The listing builds one solid part. Answer for the finished solid, in the listing's coordinates (mm). Face numbers are marked on the shaded views. A direction names the side the tool comes from. Coordinates: 2 decimals unless noted, no trailing zeros. Order: outer loops, then holes, each group sorted by start corner. A loop starts at its lowest first (then second) coordinate and runs counter-clockwise, first axis right, second up. Notation, with made-up numbers: (87, -29) -> (145, -29) arc R17 ccw to (145, -6) -> close; hole circle Ø9 at (4.5, 72.5). An arc over 180 degrees is marked (long way). Write each question's results on one line, items separated by ' | '. Start each with the question number.
(1) The part is cut by section D-D, the plane x = 6. Give the vertices of the cut face in (y, z).
(2) The part is cut by section A-A, the plane y = 0. Give the vertices of the cut face in (x, z), then the cut area to 3 significant figures.
(3) A tool of negligible diameter and unlimited length cuts with its end or side. For the marked faces 1 and 2, from which of +Z, -Z, +X, -X, +Y, -Y can it reach the whole face along a straight path? Write none if from no direction.
(4) The part is cut by section C-C, the plane z = 3.5. Give the vertices of the cut face in (x, y).
(5) Given pin 1 (1.5 mm diameter, centred on y = 5, z = -9.5, fed in from +X); pin 2 (4 mm diameter, centred on y = -4.5, z = 17.5, fed in from +X); pin 3 (3 mm diameter, centred on x = -4, z = 3.5, fed in from +Y), each flat-ended and moving along its own axis, determine where each tip first touches the part or whether it passes through.
(6) Determine the mould class of the marked faces 3 and 4 for opening direction X: +X half, -X half, draft (parallel to the pull), parting line (faces both ways), or undercut.
(7) Straight lines are drawn through the part: L1, parallel to Y at x = 0, z = -22.3; L2, parallel to Y at x = 0, z = -8; L3, parallel to Z at x = -6, y = -2.25. For each, find the intervals that lie inside material, in ascending order.
```python
from build123d import *

# Parameters (mm, degrees)
SKETCH_1_R        = 7.5
SKETCH_1_R_2      = 7
EXTRUDE_2_DEPTH   = 22.5
SKETCH_1_R_3      = 4.5
SKETCH_1_R_4      = 4
EXTRUDE_2_2_DEPTH = 22.5
SKETCH_1_5_R      = 7
SKETCH_1_5_R_2    = 4.5
EXTRUDE_3_DEPTH   = 22


with BuildPart() as part:
    # Sketch 1 → Extrude 2 (new, symmetric)
    with BuildSketch(Plane.XY):
        with Locations(Location((0, 0, 0), (0, 0, 180))):
            Circle(SKETCH_1_R)
        with Locations(Location((0, 0, 0), (0, 0, 180))):
            Circle(SKETCH_1_R_2, mode=Mode.SUBTRACT)
    extrude(amount=EXTRUDE_2_DEPTH, both=True)



with BuildPart() as body_2:
    # Sketch 1 → Extrude 2 2 (new, symmetric)
    with BuildSketch(Plane.XY):
        with Locations(Location((0, 0, 0), (0, 0, 180))):
            Circle(SKETCH_1_R_3)
        with Locations(Location((0, 0, 0), (0, 0, 180))):
            Circle(SKETCH_1_R_4, mode=Mode.SUBTRACT)
    extrude(amount=EXTRUDE_2_2_DEPTH, both=True)


with BuildPart() as part_1:
    add(part.part)

    add(body_2.part)  # Extrude 3 merges body 2
    # Sketch 1_5 → Extrude 3 (add, symmetric)
    with BuildSketch(Plane.XY):
        with Locations(Location((0, 0, 0), (0, 0, 180))):
            Circle(SKETCH_1_5_R)
        with Locations(Location((0, 0, 0), (0, 0, 180))):
            Circle(SKETCH_1_5_R_2, mode=Mode.SUBTRACT)
    extrude(amount=EXTRUDE_3_DEPTH, both=True)


solid = part_1.part
```
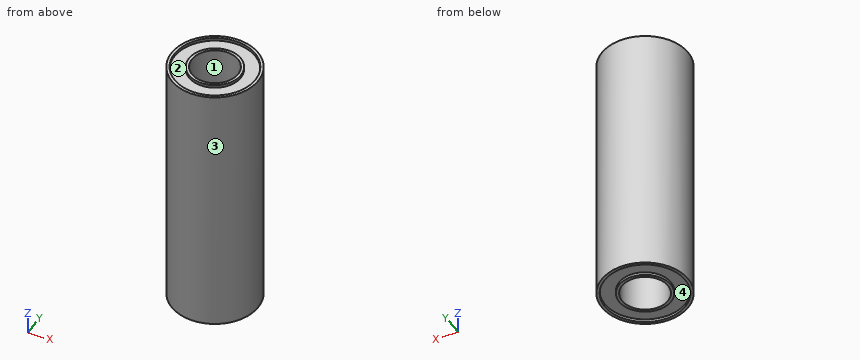
Established:
1) outline: (-4.5, -22.5) -> (-3.61, -22.5) -> (-3.61, -22) -> (3.61, -22) -> (3.61, -22.5) -> (4.5, -22.5) -> (4.5, 22.5) -> (3.61, 22.5) -> (3.61, 22) -> (-3.61, 22) -> (-3.61, 22.5) -> (-4.5, 22.5) -> close
2) outline: (-7.5, -22.5) -> (-7, -22.5) -> (-7, -22) -> (-4.5, -22) -> (-4.5, -22.5) -> (-4, -22.5) -> (-4, 22.5) -> (-4.5, 22.5) -> (-4.5, 22) -> (-7, 22) -> (-7, 22.5) -> (-7.5, 22.5) -> close; (4, -22.5) -> (4.5, -22.5) -> (4.5, -22) -> (7, -22) -> (7, -22.5) -> (7.5, -22.5) -> (7.5, 22.5) -> (7, 22.5) -> (7, 22) -> (4.5, 22) -> (4.5, 22.5) -> (4, 22.5) -> close | area: 310 mm^2
3) face 1: +Z, -Z | face 2: +Z
4) outline: circle Ø15 at (0, 0); hole circle Ø8 at (0, 0)
5) pin 1: stops at x = 6.18 | pin 2: stops at x = 7.07 | pin 3: stops at y = 7.07
6) face 3: parting line | face 4: undercut
7) L1: y = -7.5 to -7, -4.5 to -4, 4 to 4.5, 7 to 7.5 | L2: y = -7.5 to -4, 4 to 7.5 | L3: z = -22 to 22
